Source: CAD feature listing. Evaluate the final solid. Frame: model axes, mm. A direction names the side the tool comes from. Round coordinates to 2 decimals unless told otherwise and drop trailing zeros. Order: outer loops, then holes, each group sorted by start corner. A loop starts at its lowest first (then second) coordinate and runs counter-clockwise, first axis right, second up. Notation, with made-up numbers: (43.5, 89) -> (51.5, 89) arc R31 ccw to (51.5, 115) -> close; hole circle Ø6 at (-35.75, 3). An arc over 180 degrees is marked (long way). One line per item, written item: value. Start each with the question number.
1) Pin query (flat end, axial travel): P1, Ø1.8, axis at x = 16, y = 7, coming from the +Z side; P2, Ø5.5, axis at x = 3.5, z = -152.5, coming from the -Y side; P3, Ø5.5, axis at x = 18, z = -95, coming from the +Y side; P4, Ø4, axis at x = 15, y = 63, coming from the -Z side. Return the tip coordinate at first contact, or that it passes through.
2) Ray query, L1, parallel to Y at x = 2.65, z = -135; L2, parallel to X at y = 14.5, z = -42; L3, parallel to Z at x = 2.25, y = 7.5. Return the intervals inside material, ascending.
3) Mould query, pull axis Z, two halves, no side actions, for faces 1 (the face through (15, 65, -94)), 2 (the face through (3, 35, -155)), 3 (the face through (2, 60, 0)). Classes: pulls with the +Z half, pulls with the -Z half, needs draft (parallel to the pull), parting line crosses it, or undercut.
4) Reachability of faces 4 (the face through (3, 50, -152)), 5 (the face through (2, 50, 2)), 6 (the face through (15, 62, -30)) from +Z, -Z, +X, -X, +Y, -Y: full face, straight path, thin tool, end or side. Return the list, or none.
5) Section C-C (y = 40). Return the cut outline in (x, z).
6) Section A-A (x = 20). Return the cut outline in (y, z), and give its area (3 significant figures).
7) Section B-B (z = -9.5). Return the cut outline in (x, y).
Autodesk Inventor part; units mm, degrees
ref_plane "YZ Plane" through (0, 0, 0) normal (1, 0, 0) x (0, 1, 0)
ref_plane "XZ Plane" through (0, 0, 0) normal (0, 1, 0) x (-1, 0, 0)
ref_plane "XY Plane" through (0, 0, 0) normal (0, 0, 1) x (1, 0, 0)
sketch "Sketch1" plane through (0, 0, 0) normal (1, 0, 0) x (0, 1, 0)
  line L0 (0, 0) -> (70, 0)
  line L1 (70, 0) -> (70, -150)
  line L2 (70, -150) -> (0, -150)
  line L3 (0, -150) -> (0, 0)
  dimension "d0" = 70
  dimension "d1" = 150
extrude "Extrusion1" add sketch "Sketch1" along normal blind 5
sketch "Sketch2" plane through (0, 0, 0) normal (0, 0, 1) x (1, 0, 0)
  line L0 (0, 0) -> (0, 20)
  line L1 (0, 0) -> (0, 70)
  line L2 (0, 20) -> (0, 20)
  line L3 (0, 20) -> (0, 50)
  line L4 (0, 50) -> (5, 50)
  line L5 (5, 50) -> (5, 20)
  line L6 (5, 20) -> (0, 20)
  dimension "d4" = 20
  dimension "d5" = 0
  dimension "d6" = 30
  dimension "d7" = 5
extrude "Extrusion2" add sketch "Sketch2" along normal blind 5
sketch "Sketch3" plane through (0, 0, -150) normal (0, 0, -1) x (-1, 0, 0)
  line L0 (0, 0) -> (0, 0)
  line L1 (0, 0) -> (-5, 0)
  line L2 (0, 0) -> (0, 20)
  line L3 (0, 20) -> (-5, 20)
  line L4 (-5, 20) -> (-5, 50)
  line L5 (-5, 50) -> (0, 50)
  line L6 (0, 50) -> (0, 20)
  dimension "d10" = 0
  dimension "d11" = 20
  dimension "d12" = 5
  dimension "d13" = 30
extrude "Extrusion3" add sketch "Sketch3" along normal blind 5
sketch "Sketch4" plane through (5, 0, 0) normal (1, 0, 0) x (0, 0, -1)
  line L0 (0, 0) -> (150, 0)
  line L1 (0, 0) -> (0, 5)
  line L2 (0, 70) -> (0, 0)
  line L3 (0, 5) -> (28.5, 5)
  line L4 (30, 5) -> (30, 65)
  line L5 (30, 65) -> (97, 65)
  line L6 (97, 65) -> (97, 5)
  line L7 (97, 5) -> (30, 5)
  line L8 (30, 65) -> (28.5, 65)
  line L9 (28.5, 65) -> (28.5, 60)
  line L10 (28.5, 60) -> (30, 60)
  line L11 (28.5, 65) -> (28.5, 66.5)
  line L12 (28.5, 66.5) -> (35, 66.5)
  line L13 (35, 66.5) -> (35, 65)
  line L14 (28.5, 5) -> (28.5, 10)
  line L15 (28.5, 10) -> (30, 10)
  line L16 (28.5, 5) -> (28.5, 3.5)
  line L17 (28.5, 3.5) -> (35, 3.5)
  line L18 (35, 3.5) -> (35, 5)
  line L19 (97, 5) -> (98.5, 5)
  line L20 (98.5, 5) -> (98.5, 10)
  line L21 (98.5, 10) -> (97, 10)
  line L22 (98.5, 5) -> (98.5, 3.5)
  line L23 (98.5, 3.5) -> (92, 3.5)
  line L24 (92, 3.5) -> (92, 5)
  line L25 (92, 65) -> (92, 66.5)
  line L26 (92, 66.5) -> (98.5, 66.5)
  line L27 (98.5, 66.5) -> (98.5, 60)
  line L28 (98.5, 60) -> (97, 60)
  dimension "d16" = 5
  dimension "d17" = 30
  dimension "d18" = 60
  dimension "d19" = 67
  dimension "d20" = 1.5
  dimension "d21" = 5
  dimension "d22" = 1.5
  dimension "d23" = 6.5
  dimension "d24" = 5
  dimension "d25" = 1.5
  dimension "d26" = 1.5
  dimension "d27" = 5
  dimension "d28" = 1.5
  dimension "d29" = 6.5
  dimension "d30" = 6.5
  dimension "d31" = 6.5
extrude "Extrusion4" add sketch "Sketch4" along normal blind 20 contours L7 L18 L17 L16 L14 L15 L4 | L10 L9 L8 L4 | L7 L19 L22 L23 L24 | L8 L11 L12 L13 L5 | L6 L21 L20 L19 | L25 L26 L27 L28 L6 L5
fillet "Fillet1" radius 0.5 8 edges at (5, 70, -75) (0, 70, -75) (5, 0, -75) (0, 0, -75) (15, 3.5, -28.5) (15, 66.5, -28.5) (15, 66.5, -98.5) (15, 3.5, -98.5)
sketch "Sketch5" plane through (0, 0, 0) normal (-1, 0, 0) x (0, 0, 1)
  line L0 (-155, 20) -> (-155, 50)
  line L1 (-155, 35) -> (-135, 35)
  line L2 (-135, 35) -> (-135, 43.825)
  line L3 (-135, 43.825) -> (-135, 26.175)
  circle A0 centre (-135, 43.825) radius 1.025
  circle A1 centre (-135, 26.175) radius 1.025
  point P0 (0, 0)
  dimension "d35" = 20
  dimension "d36" = 8.825
  dimension "d37" = 17.65
  dimension "d38" = 2.05
  dimension "d39" = 2.05
extrude "Extrusion5" cut sketch "Sketch5" against normal through all
properties part number "Chassis_Upper_Portion"
Findings:
1. P1: z = -28.5
1. P2: y = 0
1. P3: y = 66.5
1. P4: z = -98.5
2. L1: 0 to 25.15, 27.2 to 42.8, 44.85 to 70
2. L2: 0 to 5
2. L3: -150 to 0
3. face 1: undercut
3. face 2: pulls with the -Z half
3. face 3: pulls with the +Z half
4. face 4: -Z, +X, -X, +Y
4. face 5: +Z, +X, -X, +Y
4. face 6: +X
5. outline: (0, -155) -> (5, -155) -> (5, 5) -> (0, 5) -> close
6. outline: (3.5, -98) arc R0.5 ccw to (4, -98.5) -> (10, -98.5) -> (10, -97) -> (5, -97) -> (5, -92) -> (3.5, -92) -> close; (3.5, -35) -> (5, -35) -> (5, -30) -> (10, -30) -> (10, -28.5) -> (4, -28.5) arc R0.5 ccw to (3.5, -29) -> close; (60, -98.5) -> (66, -98.5) arc R0.5 ccw to (66.5, -98) -> (66.5, -92) -> (65, -92) -> (65, -97) -> (60, -97) -> close; (60, -30) -> (65, -30) -> (65, -35) -> (66.5, -35) -> (66.5, -29) arc R0.5 ccw to (66, -28.5) -> (60, -28.5) -> close
6. area: 68.8 mm2
7. outline: (0, 0.5) arc R0.5 ccw to (0.5, 0) -> (4.5, 0) arc R0.5 ccw to (5, 0.5) -> (5, 69.5) arc R0.5 ccw to (4.5, 70) -> (0.5, 70) arc R0.5 ccw to (0, 69.5) -> close
